Here's how the part is built. I have some questions about the finished solid (model axes, mm). A direction names the side the tool comes from. Coordinates: 2 decimals unless noted, no trailing zeros. Write each loop counter-clockwise with the first axis right and the second up, starting at its lowest first coordinate (ties: lowest second). Pieces come first, ordered by that corner, then holes. Notation, with made-up numbers: (36.25, 64) -> (79.25, 64) arc R22 ccw to (79.25, 102) -> close; hole circle Ø4 at (17, 83.25). An arc over 180 degrees is marked (long way). Put each result on its own line as item: value.
```python
from build123d import *

# Parameters (mm, degrees)
BOSS_EXTRU_1_DEPTH           = 5
ESQUISSE2_R                  = 8.25
ENL_V_MAT_EXTRU_1_DEPTH      = 3
ESQUISSE4_W                  = 3
ESQUISSE4_H                  = 5
ENL_V_MAT_EXTRU_2_DEPTH      = 2
BOSS_EXTRU_2_DEPTH           = 5
ENL_V_MAT_EXTRU_4_DEPTH      = 5
ESQUISSE8_W                  = 50
ESQUISSE8_H                  = 19.6
BOSS_EXTRU_3_DEPTH           = 3
ESQUISSE10_R                 = 2.75
ENL_V_MAT_EXTRU_5_DEPTH      = 6
ENL_V_MAT_EXTRU_5_DEPTH_BACK = 9


with BuildPart() as part:
    # Esquisse1 → Boss.-Extru.1 (new body)
    with BuildSketch(Plane.XY):
        with BuildLine():
            Line((-11, -4.795831523), (-4.5, -18.795831523))
            Line((-4.5, -18.795831523), (4.5, -18.795831523))
            Line((4.5, -18.795831523), (11, -4.795831523))
            ThreePointArc((11, -4.795831523), (0, 12), (-11, -4.795831523))
        make_face()
    extrude(amount=BOSS_EXTRU_1_DEPTH)

    # Esquisse2 → Enlèv. mat.-Extru.1 (cut)
    with BuildSketch(Plane.XY.offset(5)):
        Circle(ESQUISSE2_R)
    extrude(amount=-ENL_V_MAT_EXTRU_1_DEPTH, mode=Mode.SUBTRACT)

    # Esquisse4 → Enlèv. mat.-Extru.2 (cut)
    with BuildSketch(Plane(origin=(0, 12, 0), x_dir=(1, 0, 0), z_dir=(0, 1, 0))):
        with Locations((0, -2.5)):
            Rectangle(ESQUISSE4_W, ESQUISSE4_H)
    extrude(amount=-ENL_V_MAT_EXTRU_2_DEPTH, mode=Mode.SUBTRACT)

    # Esquisse6 → Boss.-Extru.2 (add)
    with BuildSketch(Plane.XY.offset(5)):
        Polygon((0, -18.795831523), (4.5, -18.795831523), (7.75, -11.795831523), (0, -11.795831523), align=None)
    extrude(amount=BOSS_EXTRU_2_DEPTH)

    # Esquisse7 → Enlèv. mat.-Extru.4 (cut)
    with BuildSketch(Plane.XY.offset(5)):
        Polygon((0, -18.795831523), (0, -11.795831523), (-7.75, -11.795831523), (-4.5, -18.795831523), align=None)
    extrude(amount=-ENL_V_MAT_EXTRU_4_DEPTH, mode=Mode.SUBTRACT)

    # Esquisse8 → Boss.-Extru.3 (add)
    with BuildSketch(Plane(origin=(0, 0, 0), x_dir=(-1, 0, 0), z_dir=(0, 0, -1))):
        Rectangle(ESQUISSE8_W, ESQUISSE8_H)
    extrude(amount=BOSS_EXTRU_3_DEPTH)

    # Esquisse10 → Enlèv. mat.-Extru.5 (cut, two sides)
    with BuildSketch(Plane.XY.offset(5)) as enl_v_mat_extru_5_sk:
        with Locations((0, -13)):
            Circle(ESQUISSE10_R)
    extrude(amount=ENL_V_MAT_EXTRU_5_DEPTH, mode=Mode.SUBTRACT)
    extrude(enl_v_mat_extru_5_sk.sketch, amount=-ENL_V_MAT_EXTRU_5_DEPTH_BACK, mode=Mode.SUBTRACT)


solid = part.part
```
Item 1: Imagine slicing it at C-C on x = 19. Write out the boundary of the cut face in (y, z).
Output:
outline: (-9.8, -3) -> (9.8, -3) -> (9.8, 0) -> (-9.8, 0) -> close
Item 2: Please list where these lines run through material, in increasing order: line 1 along Z through (x, y) = (-5.5, 1.5); line 2 along Z through (x, y) = (18, 4.5); line 3 along Y through (x, z) = (-23, -0.25). Write a range as from..to.
Output:
line 1: z = -3..2
line 2: z = -3..0
line 3: y = -9.8..9.8
Item 3: Which directions (+Z, -Z, +X, -X, +Y, -Y) give clear straight access to the entire face, cutting with the end or side of a thin tool? Please do faces 5 (the flat face through (4, -13, 0)), 6 (the flat face through (0, 9.8, -1)), 7 (the cylindrical face through (-10.35, 6.07, 2.46)), 8 (the flat face through (0, 10, 2)), 9 (the flat face through (0, 0, 2)).
Output:
face 5: -Z, +X, -X, -Y
face 6: -Z, +X, -X, +Y
face 7: +Z, -X
face 8: +Z, -Z, +Y
face 9: +Z
Item 4: Imagine slicing it at B-B on y = 0. Write out the boundary of the cut face in (x, z), then the cut area to 4 significant figures.
Output:
outline: (-25, -3) -> (25, -3) -> (25, 0) -> (12, 0) -> (12, 5) -> (8.25, 5) -> (8.25, 2) -> (-8.25, 2) -> (-8.25, 5) -> (-12, 5) -> (-12, 0) -> (-25, 0) -> close
area: 220.5 mm²
Item 5: Imagine slicing it at D-D on y = -4. Write out the boundary of the cut face in (x, z).
Output:
outline: (-25, -3) -> (25, -3) -> (25, 0) -> (11.31, 0) -> (11.31, 5) -> (7.22, 5) -> (7.22, 2) -> (-7.22, 2) -> (-7.22, 5) -> (-11.31, 5) -> (-11.31, 0) -> (-25, 0) -> close
Item 6: Imagine slicing it at A-A on z = 3. Write out the boundary of the cut face in (x, y).
Output:
outline: (-11, -4.8) -> (-7.75, -11.8) -> (-2.47, -11.8) arc R2.75 cw (long way) to (0, -15.75) -> (0, -18.8) -> (4.5, -18.8) -> (11, -4.8) arc R12 ccw to (1.5, 11.91) -> (1.5, 10) -> (-1.5, 10) -> (-1.5, 11.91) arc R12 ccw to start; hole circle Ø16.5 at (0, 0)
Item 7: If we mould it in two halves opening along X, with no side actions, what happens to faces 1 (the flat face through (0, -17, 5)), 2 (the flat face through (0, -9.8, -1)), 3 (the cylindrical face through (2.746, -12.847, 3.959)), 4 (the flat face through (1.5, 11, 3))? For each: released by +X, released by -X, zero draft, split by the parting line, or undercut.
Output:
face 1: released by -X
face 2: zero draft
face 3: undercut
face 4: undercut
Item 8: For P1, Ø1.5, axis at x = 7, z = -1.5, coming from the -Y side; P2, Ø14.5, axis at x = -13, y = -0.5, coming from the +Z side; P3, Ø5.5, axis at x = -6.5, z = 3, coming from the -Y side, each with a flat end and sliding along its axis, tell me the tip position at first contact or that it passes through.
Output:
P1: stops at y = -9.8
P2: stops at z = 5
P3: stops at y = -11.8
